```python
from build123d import *

# Parameters (mm, degrees)
BOSS_EXTRUDE1_DEPTH = 19.05
SKETCH2_R           = 1.016
BOSS_EXTRUDE2_DEPTH = 6.35
SKETCH3_R           = 1.016
CUT_EXTRUDE1_DEPTH  = 6.35


with BuildPart() as part:
    # Sketch1 → Boss-Extrude1 (new body)
    with BuildSketch(Plane(origin=(0, 0, 0), x_dir=(1, 0, 0), z_dir=(0, 1, 0))):
        Polygon((1.3931462, -2.413), (2.786292399, 0), (1.3931462, 2.413), (-1.3931462, 2.413), (-2.786292399, 0), (-1.3931462, -2.413), align=None)
    extrude(amount=BOSS_EXTRUDE1_DEPTH)

    # Sketch2 → Boss-Extrude2 (add)
    with BuildSketch(Plane(origin=(0, 19.05, 0), x_dir=(1, 0, 0), z_dir=(0, 1, 0))):
        Circle(SKETCH2_R)
    extrude(amount=BOSS_EXTRUDE2_DEPTH)

    # Sketch3 → Cut-Extrude1 (cut)
    with BuildSketch(Plane.XZ):
        Circle(SKETCH3_R)
    extrude(amount=-CUT_EXTRUDE1_DEPTH, mode=Mode.SUBTRACT)


solid = part.part
```
Verification items for the finished model (mm, model axes). A direction names the side the tool comes from. Coordinates: 2 decimals unless noted, no trailing zeros. Loops run counter-clockwise (first coordinate to the right, second up) from the corner with the lowest first, then second, coordinate; pieces in that order, holes last. Notation, with made-up numbers: (38, 69) -> (62, 69) arc R18 cw to (62, 90) -> close; hole circle Ø4 at (63.25, 27.25). An arc over 180 degrees is marked (long way). Answer in a Markdown table with one row per item. Add a question column.
1. Section check D-D, the plane y = 12. Enter the section's corners in (x, z).
2. Section check B-B, the plane x = 0.75. Enter the section's corners in (y, z).
3. Material ranges on probe 1 along Z at (x, y) = (0, 3); probe 2 along Y at (x, z) = (1.65, 0.65); probe 3 along Y at (x, z) = (0.8, 0.55), recorded low to high. Write a range as [from, to].
4. Section check A-A, the plane y = 5.5. Enter the section's corners in (x, z).
5. Section check C-C, the plane z = 0.45. Enter the section's corners in (x, y).
6. Access from +Z, -Z, +X, -X, +Y, -Y to the whole of each face (thin tool, end or side, straight path). Record for faces 1 (the face through (-0.22, 22.18, 0.99)), 2 (the face through (2.08, 9.39, 1.22)), 3 (the face through (0, 6.35, 0)).
7. Depth check by flat-ended pin: P1, Ø2, axis at x = 2, z = -0.5, coming from the +Y side; P2, Ø1.4, axis at x = -0.5, z = 1, coming from the +Y side; P3, Ø1, axis at x = 0, z = 0, coming from the -Y side; P4, Ø1, axis at y = 9.5, z = -1, coming from the +X side. Enter the tip coordinate at first touch or a pass-through.
Derived:
| question | item | result |
|---|---|---|
| 1 | outline | (-2.79, 0) -> (-1.39, -2.41) -> (1.39, -2.41) -> (2.79, 0) -> (1.39, 2.41) -> (-1.39, 2.41) -> close |
| 2 | outline | (0, -2.41) -> (19.05, -2.41) -> (19.05, -0.69) -> (25.4, -0.69) -> (25.4, 0.69) -> (19.05, 0.69) -> (19.05, 2.41) -> (0, 2.41) -> (0, 0.69) -> (6.35, 0.69) -> (6.35, -0.69) -> (0, -0.69) -> close |
| 3 | probe 1 | z = [-2.41, -1.02], [1.02, 2.41] |
| 3 | probe 2 | y = [0, 19.05] |
| 3 | probe 3 | y = [6.35, 25.4] |
| 4 | outline | (-2.79, 0) -> (-1.39, -2.41) -> (1.39, -2.41) -> (2.79, 0) -> (1.39, 2.41) -> (-1.39, 2.41) -> close; hole circle Ø2.03 at (0, 0) |
| 5 | outline | (-2.53, 0) -> (-0.91, 0) -> (-0.91, 6.35) -> (0.91, 6.35) -> (0.91, 0) -> (2.53, 0) -> (2.53, 19.05) -> (0.91, 19.05) -> (0.91, 25.4) -> (-0.91, 25.4) -> (-0.91, 19.05) -> (-2.53, 19.05) -> close |
| 6 | face 1 | +Y |
| 6 | face 2 | +Z, +X, +Y, -Y |
| 6 | face 3 | -Y |
| 7 | P1 | stops at y = 19.05 |
| 7 | P2 | stops at y = 25.4 |
| 7 | P3 | stops at y = 6.35 |
| 7 | P4 | stops at x = 2.5 |
